```python
from build123d import *

# Parameters (mm, degrees)
BOSS_EXTRUDE1_DEPTH = 29
CUT_EXTRUDE1_REACH  = 35.231
SKETCH3_W           = 4.5
SKETCH3_H           = 1.5
CUT_EXTRUDE2_REACH  = 35.231
SKETCH4_W           = 25
SKETCH4_H           = 2.4
FILLET1_R           = 1
CHAMFER1_SIZE       = 1.75
BOSS_EXTRUDE2_DEPTH = 14
SKETCH6_W           = 2
SKETCH6_H           = 4.4
BOSS_EXTRUDE3_DEPTH = 4
CHAMFER2_SIZE       = 1
SKETCH7_W           = 100
SKETCH7_H           = 25
BOSS_EXTRUDE4_DEPTH = 2


# Some blends are built 0.0001 mm under size
with BuildPart() as part:
    # Sketch2 → Boss-Extrude1 (new body)
    with BuildSketch(Plane.XY):
        Polygon((6.559345521, 5.191043118), (9.559345521, 3.691043118), (9.559345521, 5.191043118), (9.559345521, 6.191043118), (-5.440654479, 6.191043118), (-5.440654479, 1.791043118), (9.559345521, 1.791043118), (9.559345521, 2.791043118), (-4.440654479, 2.791043118), (-4.440654479, 5.191043118), align=None)
    extrude(amount=-BOSS_EXTRUDE1_DEPTH)

    # Sketch3 → Cut-Extrude1 (cut, up to next)
    with BuildSketch(Plane(origin=(9.559345521, 0, 0), x_dir=(0, 0, -1), z_dir=(1, 0, 0)), mode=Mode.PRIVATE) as cut_extrude1_sk1:
        with Locations((2.25, 4.441043118)):
            Rectangle(SKETCH3_W, SKETCH3_H)
    cut_extrude1_tool1 = extrude(cut_extrude1_sk1.sketch, amount=-CUT_EXTRUDE1_REACH, mode=Mode.PRIVATE) & part.part
    # Sketch3 → Cut-Extrude1 (cut, up to next)
    with BuildSketch(Plane(origin=(9.559345521, 0, 0), x_dir=(0, 0, -1), z_dir=(1, 0, 0)), mode=Mode.PRIVATE) as cut_extrude1_sk2:
        with Locations((26.75, 4.441043118)):
            Rectangle(SKETCH3_W, SKETCH3_H)
    cut_extrude1_tool2 = extrude(cut_extrude1_sk2.sketch, amount=-CUT_EXTRUDE1_REACH, mode=Mode.PRIVATE) & part.part
    add(cut_extrude1_tool1.solids().sort_by_distance((9.559346, 4.441043, -2.25))[0], mode=Mode.SUBTRACT)
    add(cut_extrude1_tool2.solids().sort_by_distance((9.559346, 4.441043, -26.75))[0], mode=Mode.SUBTRACT)

    # Sketch4 → Cut-Extrude2 (cut, up to next)
    with BuildSketch(Plane.ZY.offset(5.440654479), mode=Mode.PRIVATE) as cut_extrude2_sk1:
        with Locations((-14.5, 3.991043118)):
            Rectangle(SKETCH4_W, SKETCH4_H)
    cut_extrude2_tool1 = extrude(cut_extrude2_sk1.sketch, amount=-CUT_EXTRUDE2_REACH, mode=Mode.PRIVATE) & part.part
    add(cut_extrude2_tool1.solids().sort_by_distance((-5.440654, 3.991043, -14.5))[0], mode=Mode.SUBTRACT)

    # Fillet1
    fillet1_edges = [part.edges().sort_by_distance(p)[0] for p in [
        (-5.440654479, 3.991043118, -2),
        (-5.440654479, 2.791043118, -14.5),
        (-5.440654479, 3.991043118, -27),
        (-5.440654479, 5.191043118, -14.5),
    ]]
    fillet(fillet1_edges, radius=FILLET1_R - 0.0001)  # a hair under: the kernel refuses the full size

    # Chamfer1
    # the kernel refuses this chamfer: 1.75 mm, written as the material it takes off along each edge
    with BuildSketch(Plane(origin=(14.05979075, 2.791043118, -29), x_dir=(0, -0.9996219169112968, -0.02749587661058612), z_dir=(-1, 0, 0))) as chamfer1_piece_1:
        Polygon((CHAMFER1_SIZE * 0.999621916911, CHAMFER1_SIZE * 0.0274958766106), (-CHAMFER1_SIZE * 0.0274958766106, CHAMFER1_SIZE * 0.999621916911), (0, 0), align=None)
    extrude(amount=18.500445229, mode=Mode.SUBTRACT)
    with BuildSketch(Plane(origin=(-4.440654479, 5.191043118, -29), x_dir=(0, -0.02749587661058662, 0.9996219169112968), z_dir=(1, 0, 0)), Plane(origin=(14.05979075, 5.191043118, 0), x_dir=(0, -0.02749587661058661, -0.9996219169112968), z_dir=(-1, 0, 0)), Plane(origin=(14.05979075, 2.791043118, 0), x_dir=(0, -0.9996219169112968, 0.027495876610586382), z_dir=(-1, 0, 0))) as chamfer1_piece_2:
        Polygon((CHAMFER1_SIZE * 0.999621916911, -CHAMFER1_SIZE * 0.0274958766106), (-CHAMFER1_SIZE * 0.0274958766106, -CHAMFER1_SIZE * 0.999621916911), (0, 0), align=None)
    extrude(amount=18.500445229, mode=Mode.SUBTRACT)

    # Sketch5 → Boss-Extrude2 (add)
    with BuildSketch(Plane(origin=(-4.440654479, 0, 0), x_dir=(0, 0, -1), z_dir=(1, 0, 0))):
        Polygon((0, 1.791043118), (0, 6.191043118), (0.5, 6.191043118), (1, 5.691043118), (1, 2.291043118), (0.5, 1.791043118), align=None)
        Polygon((28, 2.291043118), (28.5, 1.791043118), (29, 1.791043118), (29, 6.191043118), (28.5, 6.191043118), (28, 5.691043118), align=None)
    extrude(amount=BOSS_EXTRUDE2_DEPTH)

    # Sketch6 → Boss-Extrude3 (add)
    with BuildSketch(Plane(origin=(9.559345521, 0, 0), x_dir=(0, 0, -1), z_dir=(1, 0, 0))):
        with Locations((-1, 3.991043118)):
            Rectangle(SKETCH6_W, SKETCH6_H)
        with Locations((30, 3.991043118)):
            Rectangle(SKETCH6_W, SKETCH6_H)
    extrude(amount=-BOSS_EXTRUDE3_DEPTH)

    # Chamfer2
    chamfer2_edges = [part.edges().sort_by_distance(p)[0] for p in [
        (5.559345521, 3.991043118, 2),
        (7.559345521, 1.791043118, 2),
        (7.559345521, 6.191043118, 2),
        (9.559345521, 3.991043118, 2),
        (5.559345521, 3.991043118, -31),
        (7.559345521, 6.191043118, -31),
        (7.559345521, 1.791043118, -31),
        (9.559345521, 3.991043118, -31),
    ]]
    chamfer(chamfer2_edges, length=CHAMFER2_SIZE)

    # Sketch7 → Boss-Extrude4 (add)
    with BuildSketch(Plane(origin=(0, 6.191043118, 0), x_dir=(1, 0, 0), z_dir=(0, 1, 0))):
        with Locations((44.559345521, 14.5)):
            Rectangle(SKETCH7_W, SKETCH7_H)
    extrude(amount=BOSS_EXTRUDE4_DEPTH)


solid = part.part
```
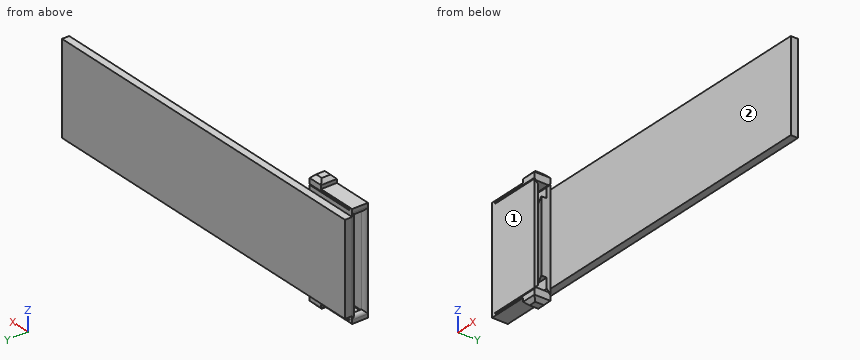
Check sheet for the modelled part. Datum: model origin and axes. Units: mm. Face numbers are marked on the shaded views. A direction names the side the tool comes from. Round coordinates to 2 decimals unless told otherwise and drop trailing zeros. Order: outer loops, then holes, each group sorted by start corner. A loop starts at its lowest first (then second) coordinate and runs counter-clockwise, first axis right, second up. Notation, with made-up numbers: (49.5, -25.75) -> (105.5, -25.75) arc R18 cw to (105.5, -12.75) -> close; hole circle Ø4 at (52.5, 28). An arc over 180 degrees is marked (long way). One line per item, written item: value. Start each with the question number.
Q1. Set-up check for the marked faces 1 and 2: record each of +Z, -Z, +X, -X, +Y, -Y from which the full face is reachable in a straight line by a thin tool's end or side.
Q2. Cross-section at A-A (x = 3.5). Record the boundary of the cut face in (y, z), and give its area (3 significant figures).
Q3. Gauge pin test, flat ends, axial feed: pin 1 Ø1.6 at (x, y) = (21, 7) entering from +Z; pin 2 Ø1.3 at (x, y) = (1, 3.5) entering from +Z; pin 3 Ø1.5 at (x, z) = (0, -29) entering from +Y. Record the tip position at first contact, or that the pin passes through.
Q4. Thickness scan on line 1 (Y direction, x = 54, z = -5.5); line 2 (Z direction, x = 36.5, y = 6.25); line 3 (X direction, y = 6, z = -23). Record the ranges inside material, lowest first.
Q5. Cross-section at D-D (x = 50). Record the boundary of the cut face in (y, z), and give its area (3 significant figures).
Completed:
1. face 1: +Z, -Z, +X, -X, -Y
1. face 2: +Z, -Z, +X, -Y
2. outline: (1.79, -29) -> (6.19, -29) -> (6.19, -28.5) -> (5.69, -28) -> (2.29, -28) -> (1.79, -28.5) -> close; (1.79, -28.25) -> (2.79, -27.25) -> (2.79, -1.75) -> (1.79, -0.75) -> close; (1.79, -0.5) -> (2.29, -1) -> (5.69, -1) -> (6.19, -0.5) -> (6.19, 0) -> (1.79, 0) -> close; (5.19, -27.25) -> (6.19, -28.25) -> (6.19, -27) -> (8.19, -27) -> (8.19, -2) -> (6.19, -2) -> (6.19, -0.75) -> (5.19, -1.75) -> close
2. area: 111 mm²
3. pin 1: stops at z = -2
3. pin 2: stops at z = 0
3. pin 3: stops at y = 6.19
4. line 1: y = 6.19 to 8.19
4. line 2: z = -27 to -2
4. line 3: x = -5.42 to 9.56
5. outline: (6.19, -27) -> (8.19, -27) -> (8.19, -2) -> (6.19, -2) -> close
5. area: 50.0 mm²
